Autodesk Inventor part; units mm, degrees
ref_plane "YZ Plane" through (0, 0, 0) normal (1, 0, 0) x (0, 1, 0)
ref_plane "XZ Plane" through (0, 0, 0) normal (0, 1, 0) x (-1, 0, 0)
ref_plane "XY Plane" through (0, 0, 0) normal (0, 0, 1) x (1, 0, 0)
sketch "Sketch1" plane through (0, 0, 0) normal (0, 0, 1) x (1, 0, 0)
  circle A0 centre (0, 0) radius 17.5
  arc A1 (21.3853, 0.9) -> (17.3853, 2) centre (15.4462, -12.8741) ccw
  arc A2 (17.3853, -2) -> (21.3853, -0.9) centre (15.4462, 12.8741) ccw
  arc A3 (21.3853, -0.9) -> (21.3853, 0.9) centre (1.4056, 0) ccw
  line L0 (0, 0) -> (21.7354, 0) construction
  arc A4 (17.3853, -2) -> (17.3853, 2) centre (0, 0) ccw
  arc A5 (19.7878, 8.1599) -> (15.6528, 7.8255) centre (18.9179, -6.8148) ccw
  arc A6 (20.4035, 6.4685) -> (19.7878, 8.1599) centre (1.3208, 0.4807) ccw
  arc A7 (17.0209, 4.0668) -> (20.4035, 6.4685) centre (10.1115, 17.3806) ccw
  circle A8 centre (0, 0) radius 17.5
  arc A9 (17.0209, 4.0668) -> (15.6528, 7.8255) centre (0, 0) ccw
  arc A10 (15.8036, 14.4357) -> (12.0324, 12.7072) centre (20.1078, 0.0665) ccw
  arc A11 (16.9606, 13.0568) -> (15.8036, 14.4357) centre (1.0768, 0.9035) ccw
  arc A12 (14.6035, 9.643) -> (16.9606, 13.0568) centre (3.5571, 19.7908) ccw
  circle A13 centre (0, 0) radius 17.5
  arc A14 (14.6035, 9.643) -> (12.0324, 12.7072) centre (0, 0) ccw
  arc A15 (9.9132, 18.9702) -> (6.9606, 16.0561) centre (18.8724, 6.9397) ccw
  arc A16 (11.4721, 18.0702) -> (9.9132, 18.9702) centre (0.7028, 1.2173) ccw
  arc A17 (10.4247, 14.0561) -> (11.4721, 18.0702) centre (-3.4262, 19.8139) ccw
  circle A18 centre (0, 0) radius 17.5
  arc A19 (10.4247, 14.0561) -> (6.9606, 16.0561) centre (0, 0) ccw
  arc A20 (2.8272, 21.2167) -> (1.0493, 17.4685) centre (15.3607, 12.976) ccw
  arc A21 (4.5999, 20.9042) -> (2.8272, 21.2167) centre (0.2441, 1.3842) ccw
  arc A22 (4.9885, 16.7739) -> (4.5999, 20.9042) centre (-9.9963, 17.4471) ccw
  circle A23 centre (0, 0) radius 17.5
  arc A24 (4.9885, 16.7739) -> (1.0493, 17.4685) centre (0, 0) ccw
  arc A25 (-4.5999, 20.9042) -> (-4.9885, 16.7739) centre (9.9963, 17.4471) ccw
  arc A26 (-2.8272, 21.2167) -> (-4.5999, 20.9042) centre (-0.2441, 1.3842) ccw
  arc A27 (-1.0493, 17.4685) -> (-2.8272, 21.2167) centre (-15.3607, 12.976) ccw
  circle A28 centre (0, 0) radius 17.5
  arc A29 (-1.0493, 17.4685) -> (-4.9885, 16.7739) centre (0, 0) ccw
  arc A30 (-11.4721, 18.0702) -> (-10.4247, 14.0561) centre (3.4262, 19.8139) ccw
  arc A31 (-9.9132, 18.9702) -> (-11.4721, 18.0702) centre (-0.7028, 1.2173) ccw
  arc A32 (-6.9606, 16.0561) -> (-9.9132, 18.9702) centre (-18.8724, 6.9397) ccw
  circle A33 centre (0, 0) radius 17.5
  arc A34 (-6.9606, 16.0561) -> (-10.4247, 14.0561) centre (0, 0) ccw
  arc A35 (-16.9606, 13.0568) -> (-14.6035, 9.643) centre (-3.5571, 19.7908) ccw
  arc A36 (-15.8036, 14.4357) -> (-16.9606, 13.0568) centre (-1.0768, 0.9035) ccw
  arc A37 (-12.0324, 12.7072) -> (-15.8036, 14.4357) centre (-20.1078, 0.0665) ccw
  circle A38 centre (0, 0) radius 17.5
  arc A39 (-12.0324, 12.7072) -> (-14.6035, 9.643) centre (0, 0) ccw
  arc A40 (-20.4035, 6.4685) -> (-17.0209, 4.0668) centre (-10.1115, 17.3806) ccw
  arc A41 (-19.7878, 8.1599) -> (-20.4035, 6.4685) centre (-1.3208, 0.4807) ccw
  arc A42 (-15.6528, 7.8255) -> (-19.7878, 8.1599) centre (-18.9179, -6.8148) ccw
  circle A43 centre (0, 0) radius 17.5
  arc A44 (-15.6528, 7.8255) -> (-17.0209, 4.0668) centre (0, 0) ccw
  arc A45 (-21.3853, -0.9) -> (-17.3853, -2) centre (-15.4462, 12.8741) ccw
  arc A46 (-21.3853, 0.9) -> (-21.3853, -0.9) centre (-1.4056, 0) ccw
  arc A47 (-17.3853, 2) -> (-21.3853, 0.9) centre (-15.4462, -12.8741) ccw
  circle A48 centre (0, 0) radius 17.5
  arc A49 (-17.3853, 2) -> (-17.3853, -2) centre (0, 0) ccw
  arc A50 (-19.7878, -8.1599) -> (-15.6528, -7.8255) centre (-18.9179, 6.8148) ccw
  arc A51 (-20.4035, -6.4685) -> (-19.7878, -8.1599) centre (-1.3208, -0.4807) ccw
  arc A52 (-17.0209, -4.0668) -> (-20.4035, -6.4685) centre (-10.1115, -17.3806) ccw
  circle A53 centre (0, 0) radius 17.5
  arc A54 (-17.0209, -4.0668) -> (-15.6528, -7.8255) centre (0, 0) ccw
  arc A55 (-15.8036, -14.4357) -> (-12.0324, -12.7072) centre (-20.1078, -0.0665) ccw
  arc A56 (-16.9606, -13.0568) -> (-15.8036, -14.4357) centre (-1.0768, -0.9035) ccw
  arc A57 (-14.6035, -9.643) -> (-16.9606, -13.0568) centre (-3.5571, -19.7908) ccw
  circle A58 centre (0, 0) radius 17.5
  arc A59 (-14.6035, -9.643) -> (-12.0324, -12.7072) centre (0, 0) ccw
  arc A60 (-9.9132, -18.9702) -> (-6.9606, -16.0561) centre (-18.8724, -6.9397) ccw
  arc A61 (-11.4721, -18.0702) -> (-9.9132, -18.9702) centre (-0.7028, -1.2173) ccw
  arc A62 (-10.4247, -14.0561) -> (-11.4721, -18.0702) centre (3.4262, -19.8139) ccw
  circle A63 centre (0, 0) radius 17.5
  arc A64 (-10.4247, -14.0561) -> (-6.9606, -16.0561) centre (0, 0) ccw
  arc A65 (-2.8272, -21.2167) -> (-1.0493, -17.4685) centre (-15.3607, -12.976) ccw
  arc A66 (-4.5999, -20.9042) -> (-2.8272, -21.2167) centre (-0.2441, -1.3842) ccw
  arc A67 (-4.9885, -16.7739) -> (-4.5999, -20.9042) centre (9.9963, -17.4471) ccw
  circle A68 centre (0, 0) radius 17.5
  arc A69 (-4.9885, -16.7739) -> (-1.0493, -17.4685) centre (0, 0) ccw
  arc A70 (4.5999, -20.9042) -> (4.9885, -16.7739) centre (-9.9963, -17.4471) ccw
  arc A71 (2.8272, -21.2167) -> (4.5999, -20.9042) centre (0.2441, -1.3842) ccw
  arc A72 (1.0493, -17.4685) -> (2.8272, -21.2167) centre (15.3607, -12.976) ccw
  circle A73 centre (0, 0) radius 17.5
  arc A74 (1.0493, -17.4685) -> (4.9885, -16.7739) centre (0, 0) ccw
  arc A75 (11.4721, -18.0702) -> (10.4247, -14.0561) centre (-3.4262, -19.8139) ccw
  arc A76 (9.9132, -18.9702) -> (11.4721, -18.0702) centre (0.7028, -1.2173) ccw
  arc A77 (6.9606, -16.0561) -> (9.9132, -18.9702) centre (18.8724, -6.9397) ccw
  circle A78 centre (0, 0) radius 17.5
  arc A79 (6.9606, -16.0561) -> (10.4247, -14.0561) centre (0, 0) ccw
  arc A80 (16.9606, -13.0568) -> (14.6035, -9.643) centre (3.5571, -19.7908) ccw
  arc A81 (15.8036, -14.4357) -> (16.9606, -13.0568) centre (1.0768, -0.9035) ccw
  arc A82 (12.0324, -12.7072) -> (15.8036, -14.4357) centre (20.1078, -0.0665) ccw
  circle A83 centre (0, 0) radius 17.5
  arc A84 (12.0324, -12.7072) -> (14.6035, -9.643) centre (0, 0) ccw
  arc A85 (20.4035, -6.4685) -> (17.0209, -4.0668) centre (10.1115, -17.3806) ccw
  arc A86 (19.7878, -8.1599) -> (20.4035, -6.4685) centre (1.3208, -0.4807) ccw
  arc A87 (15.6528, -7.8255) -> (19.7878, -8.1599) centre (18.9179, 6.8148) ccw
  circle A88 centre (0, 0) radius 17.5
  arc A89 (15.6528, -7.8255) -> (17.0209, -4.0668) centre (0, 0) ccw
  dimension "d0" = 35
  dimension "d3" = 15
  dimension "d4" = 15
  dimension "d5" = 4
  dimension "d6" = 20
  dimension "d7" = 1.8
  dimension "d10" = 360
  dimension "d20" = 2
extrude "Extrusion1" add sketch "Sketch1" along normal blind 18
sketch "Sketch2" plane through (0, 0, 18) normal (0, 0, 1) x (1, 0, 0)
  circle A0 centre (0, 0) radius 2.75
  dimension "d14" = 5.5
extrude "Extrusion2" cut sketch "Sketch2" against normal through all
sketch "Sketch5" plane through (0, 0, 0) normal (0, 1, 0) x (-1, 0, 0)
  circle A0 centre (0, 9) radius 1.4
  line L0 (2.75, 18) -> (2.75, 0)
  point P0 (0, 0)
  point P1 (2.75, 9)
  dimension "d24" = 2.8
extrude "Extrusion5" cut sketch "Sketch5" along normal through all
properties part number "BA006" material "ABS Plastic"
The model under review builds one solid part; all positions refer to its coordinate system, in mm. A direction names the side the tool comes from. Give positions to 0.01 mm unless a question says otherwise; leave off trailing zeros. Write each loop counter-clockwise with the first axis right and the second up, starting at its lowest first coordinate (ties: lowest second). Pieces come first, ordered by that corner, then holes.
1. Add section A-A, the plane x = 0. Write out the cut boundary in (y, z).
2. Add section B-B, the plane y = -5.5. Write out the cut boundary in (x, z).
3. Tool access review of faces 1 (the cylindrical face through (-11.238, -13.415, 8.874)), 2 (the cylindrical face through (-13.83, -13.69, 8.87)), 3 (the cylindrical face through (-19.395, -1.597, 8.874)), 4 (the cylindrical face through (17.237, -3.024, 8.874)): name each direction out of +Z, -Z, +X, -X, +Y, -Y from which nothing blocks a thin tool from reaching the whole face with its end or side.
4. Draft analysis for pull direction X (two halves, no side actions). For faces 5 (the cylindrical face through (19.395, 1.597, 8.874)), 6 (the cylindrical face through (-4.94, 18.82, 8.87)), 7 (the cylindrical face through (-15.917, -11.292, 8.874)), state which applies: +X half, -X half, draft (parallel to the pull), parting line (faces both ways), or undercut.
5. Wall thickness on L1, parallel to Z at x = 0, y = 14; L2, parallel to Y at x = 0, z = 4.75; L3, parallel to X at y = 18.5, z = 2.5: over which ranges is each line inside the solid? List them lowest first.
6. For P1, Ø4.5, axis at x = 0, z = 9, coming from the +Y side; P2, Ø3, axis at x = -14.5, z = 2, coming from the +Y side; P3, Ø10, axis at y = 16.5, z = 11, coming from the -X side; P4, Ø1.5, axis at x = 16, y = -9.5, coming from the +Z side, all flat-tipped, find the tip position at first contact; note any pin that passes through.
Worked answers:
1. outline: (-17.5, 0) - (-2.75, 0) - (-2.75, 18) - (-17.5, 18) - close; (2.75, 0) - (17.5, 0) - (17.5, 7.6) - (2.75, 7.6) - close; (2.75, 10.4) - (17.5, 10.4) - (17.5, 18) - (2.75, 18) - close
2. outline: (-19.27, 0) - (19.27, 0) - (19.27, 18) - (-19.27, 18) - close
3. face 1: +Z, -Z
3. face 2: +Z, -Z, -Y
3. face 3: +Z, -Z, -X
3. face 4: +Z, -Z, +X
4. face 5: +X half
4. face 6: undercut
4. face 7: -X half
5. L1: z = 0 to 7.6, 10.4 to 18
5. L2: y = -17.5 to -2.75, 2.75 to 17.5
5. L3: x = -10.77 to -9.31, -4.97 to -1.41, 1.41 to 4.97, 9.31 to 10.77
6. P1: stops at y = 20.26
6. P2: stops at y = 14.44
6. P3: stops at x = -16.96
6. P4: passes through
